Geometry check sheet. Reference: the model listing, model coordinates, mm. Coordinates: 2 decimals unless noted, no trailing zeros. Loops run counter-clockwise (first coordinate to the right, second up) from the corner with the lowest first, then second, coordinate; pieces in that order, holes last. Notation, with made-up numbers: (64, -24.75) - (109, -24.75) arc R22 cw to (109, 3.25) - close; hole circle Ø3 at (61, 81). An arc over 180 degrees is marked (long way). One line per item, written item: value.
from build123d import *

# Parameters (mm, degrees)
SKETCH1_R           = 5.5
SKETCH1_R_2         = 2.5
BOSS_EXTRUDE1_DEPTH = 5
SKETCH2_R           = 3.6
SKETCH2_R_2         = 3.4
CUT_EXTRUDE1_DEPTH  = 0.1
CUT_EXTRUDE2_START  = -0.1
SKETCH3_R           = 3.8
SKETCH3_R_2         = 3.4
CUT_EXTRUDE2_DEPTH  = 0.1


with BuildPart() as part:
    # Sketch1 → Boss-Extrude1 (new body)
    with BuildSketch(Plane.XY):
        Circle(SKETCH1_R)
        Circle(SKETCH1_R_2, mode=Mode.SUBTRACT)
    extrude(amount=BOSS_EXTRUDE1_DEPTH)

    # Sketch2 → Cut-Extrude1 (cut)
    with BuildSketch(Plane.XY.offset(5)):
        Circle(SKETCH2_R)
        Circle(SKETCH2_R_2, mode=Mode.SUBTRACT)
    extrude(amount=-CUT_EXTRUDE1_DEPTH, mode=Mode.SUBTRACT)

    # Sketch3 → Cut-Extrude2 (cut)
    with BuildSketch(Plane(origin=(0, 0, 0), x_dir=(-1, 0, 0), z_dir=(0, 0, -1)).offset(CUT_EXTRUDE2_START)):
        Circle(SKETCH3_R)
        with Locations(Location((0, 0, 0), (0, 0, 180))):
            Circle(SKETCH3_R_2, mode=Mode.SUBTRACT)
    extrude(amount=CUT_EXTRUDE2_DEPTH, mode=Mode.SUBTRACT)


solid = part.part
(1) Cross-section at D-D on y = -4.25. Record the cut outline in (x, z).
Reply:
outline: (-3.49, 0) - (3.49, 0) - (3.49, 5) - (-3.49, 5) - close
(2) Go/stop test with flat-tipped pins: pin 1 Ø6 at (x, y) = (0, 0) entering from +Z; pin 2 Ø3 at (y, z) = (4, 4) entering from -X; pin 3 Ø2 at (x, z) = (-2.5, 2) entering from +Y. Record where each tip stops, or that it passes through.
Reply:
pin 1: z = 5
pin 2: x = -4.9
pin 3: y = 5.29
(3) Cross-section at C-C on z = 2.8. Record the cut outline in (x, y), and give its area (3 significant figures).
Reply:
outline: circle Ø11 at (0, 0); hole circle Ø5 at (0, 0)
area: 75.4 mm2
(4) Cross-section at A-A on y = 0. Record the cut outline in (x, z).
Reply:
outline: (-5.5, 0) - (-3.8, 0) - (-3.8, 0.1) - (-3.4, 0.1) - (-3.4, 0) - (-2.5, 0) - (-2.5, 5) - (-3.4, 5) - (-3.4, 4.9) - (-3.6, 4.9) - (-3.6, 5) - (-5.5, 5) - close; (2.5, 0) - (3.4, 0) - (3.4, 0.1) - (3.8, 0.1) - (3.8, 0) - (5.5, 0) - (5.5, 5) - (3.6, 5) - (3.6, 4.9) - (3.4, 4.9) - (3.4, 5) - (2.5, 5) - close
(5) Release check for a two-part mould opening along Y. For faces 1 (the face through (-1.19, -5.37, 2.46)), 2 (the face through (-0.54, -2.44, 2.46)), 3 (the face through (3, -2, 0.1)), 4 (the face through (-2, 2, 5)) record: pulls with the +Y half, pulls with the -Y half, needs draft (parallel to the pull), parting line crosses it, or undercut.
Reply:
face 1: parting line crosses it
face 2: undercut
face 3: undercut
face 4: needs draft
(6) Material ranges on probe 1 along Y at (x, z) = (0, 4.95); probe 2 along Y at (x, z) = (0, 0.15); probe 3 along X at (y, z) = (2, 4.5), recorded low to high. Write a range as from..to.
Reply:
probe 1: -5.5..-3.6, -3.4..-2.5, 2.5..3.4, 3.6..5.5
probe 2: -5.5..-2.5, 2.5..5.5
probe 3: -5.12..-1.5, 1.5..5.12
